Can you work these out from the model? Positions are in its coordinate system, mm. A direction names the side the tool comes from. Give positions to 0.01 mm unless a question says otherwise; leave off trailing zeros. Loops run counter-clockwise (first coordinate to the right, second up) from the corner with the lowest first, then second, coordinate; pieces in that order, holes last. Notation, with made-up numbers: (-6.75, -4) - (4.25, -4) arc R18 cw to (4.25, 20) - close; hole circle Ø6 at (62, -10). An arc over 180 degrees is marked (long way). Answer in a Markdown table with one row per item.
from build123d import *

# Parameters (mm, degrees)
SKETCH_1_W          = 70
SKETCH_1_H          = 100
EXTRUDE_1_DEPTH     = 40
SKETCH_2_W          = 50.2
SKETCH_2_H          = 100
CUT_EXTRUDE_1_DEPTH = 36
CUT_EXTRUDE_2_REACH = 130.452
SKETCH_3_R          = 1.5
CUT_EXTRUDE_4_REACH = 129.264
SKETCH_6_R          = 0.799974648
SKETCH_6_R_2        = 0.799973527
SKETCH_6_R_3        = 0.799971754
SKETCH_6_R_4        = 0.799972464


with BuildPart() as part:
    # 草图1 → 凸台-拉伸1 (new body)
    with BuildSketch(Plane.XY):
        with Locations((35, 50)):
            Rectangle(SKETCH_1_W, SKETCH_1_H)
    extrude(amount=EXTRUDE_1_DEPTH)

    # 草图2 → 切除-拉伸1 (cut)
    with BuildSketch(Plane.XY.offset(40)):
        with Locations((35, 50)):
            Rectangle(SKETCH_2_W, SKETCH_2_H)
    extrude(amount=-CUT_EXTRUDE_1_DEPTH, mode=Mode.SUBTRACT)

    # 草图3 → 切除-拉伸2 (cut, up to next)
    with BuildSketch(Plane(origin=(0, 0, 0), x_dir=(-1, 0, 0), z_dir=(0, 0, -1)), mode=Mode.PRIVATE) as cut_extrude_2_sk1:
        with Locations((-35, 50)):
            Circle(SKETCH_3_R)
    cut_extrude_2_tool1 = extrude(cut_extrude_2_sk1.sketch, amount=-CUT_EXTRUDE_2_REACH, mode=Mode.PRIVATE) & part.part
    add(cut_extrude_2_tool1.solids().sort_by_distance((35, 50, 0))[0], mode=Mode.SUBTRACT)

    # 草图6 → 切除-拉伸4 (cut, up to next)
    with BuildSketch(Plane.XY.offset(4), mode=Mode.PRIVATE) as cut_extrude_4_sk1:
        with Locations((35.098154463, 42.913706308)):
            Circle(SKETCH_6_R)
    cut_extrude_4_tool1 = extrude(cut_extrude_4_sk1.sketch, amount=-CUT_EXTRUDE_4_REACH, mode=Mode.PRIVATE) & part.part
    # 草图6 → 切除-拉伸4 (cut, up to next)
    with BuildSketch(Plane.XY.offset(4), mode=Mode.PRIVATE) as cut_extrude_4_sk2:
        with Locations((28.096062907, 49.911346021)):
            Circle(SKETCH_6_R_2)
    cut_extrude_4_tool2 = extrude(cut_extrude_4_sk2.sketch, amount=-CUT_EXTRUDE_4_REACH, mode=Mode.PRIVATE) & part.part
    # 草图6 → 切除-拉伸4 (cut, up to next)
    with BuildSketch(Plane.XY.offset(4), mode=Mode.PRIVATE) as cut_extrude_4_sk3:
        with Locations((35.09343748, 56.91370551)):
            Circle(SKETCH_6_R_3)
    cut_extrude_4_tool3 = extrude(cut_extrude_4_sk3.sketch, amount=-CUT_EXTRUDE_4_REACH, mode=Mode.PRIVATE) & part.part
    # 草图6 → 切除-拉伸4 (cut, up to next)
    with BuildSketch(Plane.XY.offset(4), mode=Mode.PRIVATE) as cut_extrude_4_sk4:
        with Locations((42.095529036, 49.916065797)):
            Circle(SKETCH_6_R_4)
    cut_extrude_4_tool4 = extrude(cut_extrude_4_sk4.sketch, amount=-CUT_EXTRUDE_4_REACH, mode=Mode.PRIVATE) & part.part
    add(cut_extrude_4_tool1.solids().sort_by_distance((35.098154, 42.913706, 4))[0], mode=Mode.SUBTRACT)
    add(cut_extrude_4_tool2.solids().sort_by_distance((28.096063, 49.911346, 4))[0], mode=Mode.SUBTRACT)
    add(cut_extrude_4_tool3.solids().sort_by_distance((35.093437, 56.913706, 4))[0], mode=Mode.SUBTRACT)
    add(cut_extrude_4_tool4.solids().sort_by_distance((42.095529, 49.916066, 4))[0], mode=Mode.SUBTRACT)


solid = part.part
Q1. For pin 1 (2 mm diameter, centred on x = 35.09, y = 56.91, fed in from -Z); pin 2 (2.5 mm diameter, centred on x = 42.1, y = 49.92, fed in from +Z), each with a flat end and sliding along its axis, tell me the tip position at first contact or that it passes through.
Checked values:
| item | result |
|---|---|
| pin 1 | stops at z = 0 |
| pin 2 | stops at z = 4 |
Q2. Imagine slicing it at B-B, the plane y = 12.5. Write out the boundary of the cut face in (x, z).
Checked values:
| item | result |
|---|---|
| outline | (0, 0) - (70, 0) - (70, 40) - (60.1, 40) - (60.1, 4) - (9.9, 4) - (9.9, 40) - (0, 40) - close |
Q3. On a 3-axis mill with a long thin cutter (end or side, diameter ignored), from which of +Z, -Z, +X, -X, +Y, -Y can I reach the whole of each face in a straight line? I mean faces 4 (the face through (9.9, 49, 22)), 5 (the face through (42, 51, 0)). Say none if no direction works.
Checked values:
| item | result |
|---|---|
| face 4 | +Z, +Y, -Y |
| face 5 | -Z, +X, -X, +Y, -Y |
Q4. If we mould it in two halves opening along X, with no side actions, what happens to faces 1 (the face through (0, 49, 20)), 2 (the face through (35.325, 48.536, 1.972)), 3 (the face through (65, 51, 40))? For each: released by +X, released by -X, zero draft, split by the parting line, or undercut.
Checked values:
| item | result |
|---|---|
| face 1 | released by -X |
| face 2 | undercut |
| face 3 | zero draft |
Q5. If I drill on line 1 (Y direction, x = 35, z = 3.5); line 2 (X direction, y = 86, z = 15.5); line 3 (Z direction, x = 54, y = 88), over which ranges is the centre line in solid material (lowest first)? Write a range as [from, to].
Checked values:
| item | result |
|---|---|
| line 1 | y = [0, 42.12], [43.71, 48.5], [51.5, 56.12], [57.71, 100] |
| line 2 | x = [0, 9.9], [60.1, 70] |
| line 3 | z = [0, 4] |
Q6. Imagine slicing it at C-C, the plane x = 15.5. Write out the boundary of the cut face in (y, z), and give its area (3 significant figures).
Checked values:
| item | result |
|---|---|
| outline | (0, 0) - (100, 0) - (100, 4) - (0, 4) - close |
| area | 400 mm² |
Q7. Imagine slicing it at A-A, the plane z = 10.5. Write out the boundary of the cut face in (x, y).
Checked values:
| item | result |
|---|---|
| outline | (0, 0) - (9.9, 0) - (9.9, 100) - (0, 100) - close; (60.1, 0) - (70, 0) - (70, 100) - (60.1, 100) - close |
